Verification items for the finished model (mm, model axes). A direction names the side the tool comes from. Round coordinates to 2 decimals unless told otherwise and drop trailing zeros. Loops run counter-clockwise (first coordinate to the right, second up) from the corner with the lowest first, then second, coordinate; pieces in that order, holes last. Notation, with made-up numbers: M -31.5,19 L 5.5,19 A21 ccw 5.5,32 Z; hole C -17.75,78.5 d7. An arc over 180 degrees is marked long. One line per item, written item: value.
Autodesk Inventor part; units mm, degrees
ref_plane "YZ Plane" through (0, 0, 0) normal (1, 0, 0) x (0, 1, 0)
ref_plane "XZ Plane" through (0, 0, 0) normal (0, 1, 0) x (-1, 0, 0)
ref_plane "XY Plane" through (0, 0, 0) normal (0, 0, 1) x (1, 0, 0)
sketch "Sketch1" plane through (0, 0, 0) normal (0, 1, 0) x (-1, 0, 0)
  line L0 (20, -15.715) -> (-20, -15.715)
  line L1 (-20, -15.715) -> (-20, 15.715)
  line L2 (-20, 15.715) -> (20, 15.715)
  line L3 (20, 15.715) -> (20, -15.715)
  point P0 (0, 0)
  dimension "d0" = 40
  dimension "d1" = 20
  dimension "d2" = 31.43
  dimension "d3" = 15.715
extrude "Plate1" add sketch "Sketch1" along normal blind 1.5
sketch "Sketch2" plane through (20, 0, 17.215) normal (0, 0, -1) x (-1, 0, 0)
  line L0 (40, 0) -> (0, 0)
  line L1 (0, 0) -> (0, 45)
  line L2 (0, 45) -> (40, 45)
  line L3 (40, 45) -> (40, 0)
edge flange "Flange1" height 45 angle 90 thickness 1.5 bend radius 0.31 thickness toward (0, 0, -1) relief tear relief width 1.5 relief depth 0.75 edges at (0, 1.5, 15.715) wall of the first edge with corners at (-20, 0, 17.215) (20, 0, 17.215) (20, 45, 17.215) (-20, 45, 17.215)
bend "Bend1"
corner "Corner1"
sketch "Sketch3" plane through (-20, 0, -17.215) normal (0, 0, 1) x (1, 0, 0)
  line L0 (40, 0) -> (0, 0)
  line L1 (0, 0) -> (0, 45)
  line L2 (0, 45) -> (40, 45)
  line L3 (40, 45) -> (40, 0)
edge flange "Flange2" height 45 angle 90 thickness 1.5 bend radius 0.31 thickness toward (0, 0, 1) relief tear relief width 1.5 relief depth 0.75 edges at (0, 1.5, -15.715) wall of the first edge with corners at (20, 0, -17.215) (-20, 0, -17.215) (-20, 45, -17.215) (20, 45, -17.215)
bend "Bend2"
corner "Corner2"
sketch "Sketch4" plane through (-20, 45, 17.215) normal (0, 0, 1) x (1, 0, 0)
  line L0 (0, -43.19) -> (0, 0)
  line L1 (0, 0) -> (40, 0)
  line L2 (40, 0) -> (40, -43.19)
  line L3 (0, -43.19) -> (40, -43.19)
  arc A0 (28.9876, -5.6156) -> (11.0124, -5.6156) centre (20, -10) ccw
  line L4 (0, -38.19) -> (40, -38.19)
  line L5 (40, -38.19) -> (40, -28.19)
  line L6 (40, -28.19) -> (0, -28.19)
  line L7 (0, -28.19) -> (0, -38.19)
  line L8 (40, -28.19) -> (28.9876, -5.6156)
  line L9 (11.0124, -5.6156) -> (0, -28.19)
  point P0 (0, -28.19)
  point P1 (20, 0)
  point P2 (40, -28.19)
  dimension "d50" = 10
  dimension "d51" = 20
  dimension "d52" = 20
  dimension "d53" = 38.19
  dimension "d54" = 10
  dimension "d55" = 40
  dimension "d56" = 40
extrude "Extrusion1" cut sketch "Sketch4" against normal blind 50 contours L0 L1 A0 L9 | L8 A0 L1 L2
sketch "Sketch5" plane through (20, 1.81, -17.215) normal (0, 0, -1) x (-1, 0, 0)
  arc A0 (20, 38.19) -> (20, 38.19) centre (20, 28.19) ccw
  circle A1 centre (20, 35.19) radius 1.05
  circle A2 centre (13, 28.19) radius 1.05
  circle A3 centre (20, 21.19) radius 1.05
  circle A4 centre (27, 28.19) radius 1.05
  point P0 (20, -1.81)
  dimension "d36" = 7
  dimension "d37" = 0
  dimension "d38" = 2.1
  dimension "d41" = 360
hole "Hole1" at (7, 30, -17.215) at (0, 23, -17.215) at (-7, 30, -17.215) at (0, 37, -17.215) direction (0, 0, 1) diameter 2.1 depth 1.5
sketch "Sketch6" plane through (-20, 1.81, 17.215) normal (0, 0, 1) x (1, 0, 0)
  arc A0 (28.9876, 37.5744) -> (11.0124, 37.5744) centre (20, 33.19) ccw
  point P0 (20, -1.81)
hole "Hole2" at (0, 35, 17.215) direction (0, 0, -1) diameter 3 depth 1.5
sketch "Sketch7" plane through (-20, 1.81, -15.715) normal (0, 0, 1) x (1, 0, 0)
  arc A0 (28.9876, 37.5744) -> (11.0124, 37.5744) centre (20, 33.19) ccw
  point P0 (20, -1.81)
hole "Hole3" at (0, 35, -15.715) direction (0, 0, -1) diameter 5.2 depth 1.5
sketch "Sketch8" plane through (0, 1.5, 0) normal (0, 1, 0) x (1, 0, 0)
  line L0 (20, 15.405) -> (20, -15.405)
  line L1 (20, -15.715) -> (-20, -15.715)
  line L2 (-20, -15.405) -> (20, -15.405)
  line L3 (20, 15.405) -> (-20, 15.405)
  point P0 (0, 0)
  point P1 (14, -9.405)
  point P2 (-14, -9.405)
  point P3 (14, 0)
  point P4 (-14, 0)
  point P5 (14, 9.405)
  point P6 (-14, 9.405)
  dimension "d71" = 6
  dimension "d73" = 6
  dimension "d76" = 28
  dimension "d79" = 9.405
hole "Hole4" at (14, 1.5, 9.405) at (-14, 1.5, 9.405) at (14, 1.5, 0) at (-14, 1.5, 0) at (14, 1.5, -9.405) at (-14, 1.5, -9.405) direction (0, -1, 0) diameter 2.1 depth 1.5
equation "\"d48\" = Thickness"
equation "\"d62\" = Thickness"
equation "\"d69\" = Thickness"
equation "\"d87\" = Thickness"
equation "\"d4\" = Thickness"
equation "\"d5\" = BendReliefWidth"
equation "\"d6\" = BendReliefDepth"
equation "\"d7\" = MinimumRemnant"
equation "\"d8\" = TransitionRadius"
equation "\"d11\" = BendRadius"
equation "\"d12\" = CornerReliefSize"
equation "\"d13\" = GapSize"
equation "\"d14\" = JacobiRadiusSize"
equation "\"d15\" = BendReliefWidth"
equation "\"d16\" = BendReliefDepth"
equation "\"d17\" = MinimumRemnant"
equation "\"d18\" = TransitionRadius"
equation "\"d21\" = BendRadius"
equation "\"d22\" = CornerReliefSize"
equation "\"d23\" = GapSize"
equation "\"d24\" = JacobiRadiusSize"
equation "\"BendReliefWidth\" = Thickness"
equation "\"BendReliefDepth\" = 0.5 * Thickness"
equation "\"CornerReliefSize\" = 4 * Thickness"
equation "\"MinimumRemnant\" = 2 * Thickness"
equation "\"TransitionRadius\" = BendRadius"
equation "\"JacobiRadiusSize\" = BendRadius"
equation "\"GapSize\" = Thickness"
properties part number "axis_12_bottom_frame(top)" material "Aluminum 6061-AHC"
(1) Tool access check on faces 1 (the face through (0, 18, 15.715)), 2 (the face through (0.9, 36.2, 16.5)), 3 (the face through (6.68, 31, -16.45)). Record the directions out of +Z, -Z, +X, -X, +Y, -Y that give a thin tool (end or side, any length) a straight path to the whole face; none if there is none.
Completed:
face 1: +X, -X, +Y
face 2: +Z, -Z
face 3: -Z
(2) Mould release check, pull along Y, two halves, no side actions. Record for faces 4 (the face through (0.02, 38.05, -16.45)), 5 (the face through (-0.28, 0.544, -16.699)), 6 (the face through (14.57, 27.94, 16.48)): +Y half, -Y half, draft (parallel to the pull), parting line (faces both ways), or undercut.
Completed:
face 4: undercut
face 5: -Y half
face 6: +Y half
(3) Sectioned sample at D-D on y = 23. Enter the section's corners in (x, z) (3 decimals).
Completed:
outline: M -16.98,-17.215 L -1.05,-17.215 L -1.05,-15.715 L -16.98,-15.715 Z; M -16.98,15.715 L 16.98,15.715 L 16.98,17.215 L -16.98,17.215 Z; M 1.05,-17.215 L 16.98,-17.215 L 16.98,-15.715 L 1.05,-15.715 Z
(4) Sectioned sample at B-B on z = 0. Enter the section's corners in (x, y).
Completed:
outline: M -20,0 L -15.05,0 L -15.05,1.5 L -20,1.5 Z; M -12.95,0 L 12.95,0 L 12.95,1.5 L -12.95,1.5 Z; M 15.05,0 L 20,0 L 20,1.5 L 15.05,1.5 Z
(5) Depth check by flat-ended pin: pin 1 Ø3.5 at (x, z) = (14, -9.405) entering from +Y; pin 2 Ø1.9 at (x, y) = (-7, 30) entering from -Z (3 decimals). Enter the tip coordinate at first touch or a pass-through.
Completed:
pin 1: stops at y = 1.5
pin 2: stops at z = 15.715
(6) Thickness scan on L1, parallel to Z at x = 14, y = 0.85 (3 decimals); L2, parallel to Z at x = -6, y = 3 (3 decimals); L3, parallel to Y at x = 1.5, z = -2. Record the ranges inside material, lowest first. Write a range as from..to.
Completed:
L1: z = -16.939..-10.455, -8.355..-1.05, 1.05..8.355, 10.455..16.939
L2: z = -17.215..-15.715, 15.715..17.215
L3: y = 0..1.5
(7) Sectioned sample at A-A on y = 14.5. Enter the section's corners in (x, z) (3 decimals).
Completed:
outline: M -20,-17.215 L 20,-17.215 L 20,-15.715 L -20,-15.715 Z; M -20,15.715 L 20,15.715 L 20,17.215 L -20,17.215 Z
(8) Sectioned sample at C-C on x = 0. Enter the section's corners in (y, z) (3 decimals).
Completed:
outline: M 0,-15.405 A1.81 ccw 1.81,-17.215 L 21.95,-17.215 L 21.95,-15.715 L 1.81,-15.715 A0.31 cw 1.5,-15.405 L 1.5,15.405 A0.31 cw 1.81,15.715 L 33.5,15.715 L 33.5,17.215 L 1.81,17.215 A1.81 ccw 0,15.405 Z; M 24.05,-17.215 L 32.4,-17.215 L 32.4,-15.715 L 24.05,-15.715 Z; M 36.5,15.715 L 45,15.715 L 45,17.215 L 36.5,17.215 Z; M 38.05,-17.215 L 45,-17.215 L 45,-15.715 L 38.05,-15.715 Z
